Autodesk Inventor part; units mm, degrees
ref_plane "YZ Plane" through (0, 0, 0) normal (1, 0, 0) x (0, 1, 0)
ref_plane "XZ Plane" through (0, 0, 0) normal (0, 1, 0) x (-1, 0, 0)
ref_plane "XY Plane" through (0, 0, 0) normal (0, 0, 1) x (1, 0, 0)
sketch "スケッチ1" plane through (0, 0, 0) normal (0, 0, 1) x (1, 0, 0)
  line L0 (0, 0) -> (0, 23.3181) construction
  line L1 (-22.6457, 22) -> (22.6457, 22) construction
  line L2 (-20.3832, 1.5) -> (20.3832, 1.5) construction
  circle A0 centre (0, 22) radius 14 construction
  line L3 (-22.6457, 14) -> (22.6457, 14) construction
  circle A1 centre (-17.5, 22) radius 2.1
  circle A2 centre (17.5, 22) radius 2.1
  line L4 (-21.5, 26) -> (-21.5, 0)
  line L5 (-21.5, 0) -> (-14.25, 0)
  line L6 (-14.25, 0) -> (-14.25, 26)
  line L7 (21.5, 26) -> (21.5, 0)
  line L8 (21.5, 0) -> (14.25, 0)
  line L9 (14.25, 0) -> (14.25, 26)
  line L10 (-14.25, 26) -> (-21.5, 26)
  line L11 (14.25, 26) -> (21.5, 26)
  line L12 (21.5, 1.5) -> (-21.5, 1.5)
  line L13 (-21.5, 1.5) -> (-21.5, 0)
  line L14 (-21.5, 0) -> (21.5, 0)
  line L15 (21.5, 0) -> (21.5, 1.5)
  point P0 (0, 1.5)
  point P1 (0, 14)
  point P2 (14.25, 1.5)
  point P3 (-14.25, 1.5)
  point P4 (0, 0)
  dimension "d0" = 28
  dimension "d1" = 1.5
  dimension "d2" = 8
  dimension "d3" = 4.2
  dimension "d4" = 35
  dimension "d29" = 3.25
  dimension "d30" = 3.25
  dimension "d31" = 4
  dimension "d32" = 4
  dimension "d46" = 22
  dimension "d47" = 4
extrude "前" add sketch "スケッチ1" along normal blind 2
extrude "底" add sketch "スケッチ1" against normal blind 15 contours L12 L6 L5 L4 | L12 L9 L14 L6 | L12 L7 L8 L9
sketch "スケッチ5" plane through (-14.25, 1.5, 2) normal (0, 1, 0) x (1, 0, 0)
  line L0 (14.25, -6.214) -> (14.25, 25.3742) construction
  line L1 (28.5, 0) -> (0, 0) construction
  point P0 (14.25, 2)
  point P1 (-3.25, 14)
  point P2 (31.75, 14)
  dimension "d33" = 35
  dimension "d34" = 14
hole "穴2" at (-17.5, 1.5, -12) at (17.5, 1.5, -12) direction (0, -1, 0) diameter 3.2 end through all
sketch "スケッチ6" plane through (21.5, 1.5, 0) normal (1, 0, 0) x (0, 0, -1)
  line L0 (2, 24.5) -> (-2, 24.5)
  line L1 (-2, 24.5) -> (-2, 0)
  line L2 (-2, 24.5) -> (-2, -1.5)
  line L3 (-2, -1.5) -> (8, -1.5)
  line L4 (8, -1.5) -> (8, 0)
  line L5 (8, 0) -> (2, 24.5)
  point P0 (0, -1.5)
  point P1 (15, 0)
  dimension "d42" = 4
  dimension "d43" = 10
extrude "押し出し5" add sketch "スケッチ6" along normal blind 0.8
mirror "ミラー3" about plane through (0, 0, 0) normal (1, 0, 0) of "押し出し5"
equation "\"d30\" = d29"
equation "\"d32\" = d31"
properties part number "28BYJ-48_Braket3"
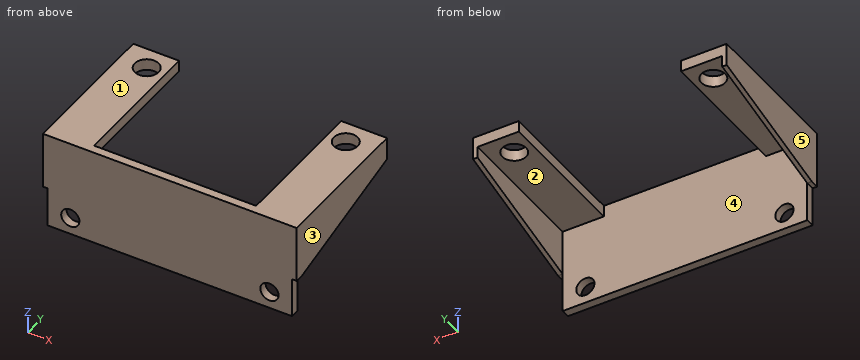
Here's how the part is built. I have some questions about the finished solid (model axes, mm). Face numbers are marked on the shaded views. A direction names the side the tool comes from. Give positions to 0.01 mm unless a question says otherwise; leave off trailing zeros. Loops run counter-clockwise (first coordinate to the right, second up) from the corner with the lowest first, then second, coordinate; pieces in that order, holes last. Notation, with made-up numbers: (42, 25) -> (79, 25) arc R29 ccw to (79, 47) -> close; hole circle Ø3 at (40, 37.25). An arc over 180 degrees is marked (long way). Answer as a JSON object with one key per item and string values. Group by question number.
Item 1: Thinking about a two-plate mould opening in X: for the marked faces 3, 4 and 5, which applies, pulls with the +X half, pulls with the -X half, needs draft (parallel to the pull), parting line crosses it, or undercut?
Item 2: On a 3-axis mill with a long thin cutter (end or side, diameter ignored), from which of +Z, -Z, +X, -X, +Y, -Y can I reach the whole of each face in a straight line? I mean the marked faces 1 and 2. Say none if no direction works.
Item 3: Will these pins go through, and if not, where does the flat tip stop? pin 1 (1.9 mm diameter, centred on x = -17.5, z = -12, fed in from -Y); pin 2 (3.5 mm diameter, centred on x = 17, y = 19.5, fed in from -Z); pin 3 (8 mm diameter, centred on x = 8, z = -6, fed in from +Y); pin 4 (1.2 mm diameter, centred on y = 1, z = -11.5, fed in from -X).
Item 4: Imagine slicing it at A-A on z = -12. Write out the boundary of the cut face in (x, y).
Item 5: Imagine slicing it at B-B on x = -17.5. Write out the boundary of the cut face in (y, z), then the cut area to 3 significant figures.
Item 6: Imagine slicing it at D-D on z = 1. Write out the boundary of the cut face in (x, y), then the cut area to 3 significant figures.
Item 7: I need wall thicknesses on L1, parallel to X at y = 1.05, z = -12; L2, parallel to Y at x = -17.5, z = 1.5; L3, parallel to X at y = 18, z = -0.5. Which ranges of each line are inside material? Lowest first, please.
Item 8: Imagine slicing it at C-C on y = 7. Write out the boundary of the cut face in (x, z), then the cut area to 3 significant figures.
Answer list:
{
 "1": {"face 3": "pulls with the +X half", "face 4": "undercut", "face 5": "pulls with the -X half"},
 "2": {"face 1": "+Z, +X, -X, +Y, -Y", "face 2": "-Z, +Y"},
 "3": {"pin 1": "passes through", "pin 2": "stops at z = 0", "pin 3": "stops at y = 1.5", "pin 4": "stops at x = -21.5"},
 "4": {"outline": "(-21.5, 0) -> (-19.1, 0) -> (-19.1, 1.5) -> (-21.5, 1.5) -> close; (-15.9, 0) -> (15.9, 0) -> (15.9, 1.5) -> (-15.9, 1.5) -> close; (19.1, 0) -> (21.5, 0) -> (21.5, 1.5) -> (19.1, 1.5) -> close"},
 "5": {"outline": "(0, -15) -> (1.5, -15) -> (1.5, -13.6) -> (0, -13.6) -> close; (0, -10.4) -> (1.5, -10.4) -> (1.5, 0) -> (19.9, 0) -> (19.9, 2) -> (0, 2) -> close; (24.1, 0) -> (26, 0) -> (26, 2) -> (24.1, 2) -> close", "area": "61.3 mm2"},
 "6": {"outline": "(-22.3, 0) -> (22.3, 0) -> (22.3, 26) -> (14.25, 26) -> (14.25, 1.5) -> (-14.25, 1.5) -> (-14.25, 26) -> (-22.3, 26) -> close; hole circle Ø4.2 at (-17.5, 22); hole circle Ø4.2 at (17.5, 22)", "area": "434 mm2"},
 "7": {"L1": "x = -21.5 to -19.1, -15.9 to 15.9, 19.1 to 21.5", "L2": "y = 0 to 19.9, 24.1 to 26", "L3": "x = -22.3 to -21.5, 21.5 to 22.3"},
 "8": {"outline": "(-22.3, -6.65) -> (-21.5, -6.65) -> (-21.5, 0) -> (-14.25, 0) -> (-14.25, 2) -> (-22.3, 2) -> close; (14.25, 0) -> (21.5, 0) -> (21.5, -6.65) -> (22.3, -6.65) -> (22.3, 2) -> (14.25, 2) -> close", "area": "42.8 mm2"}
}
